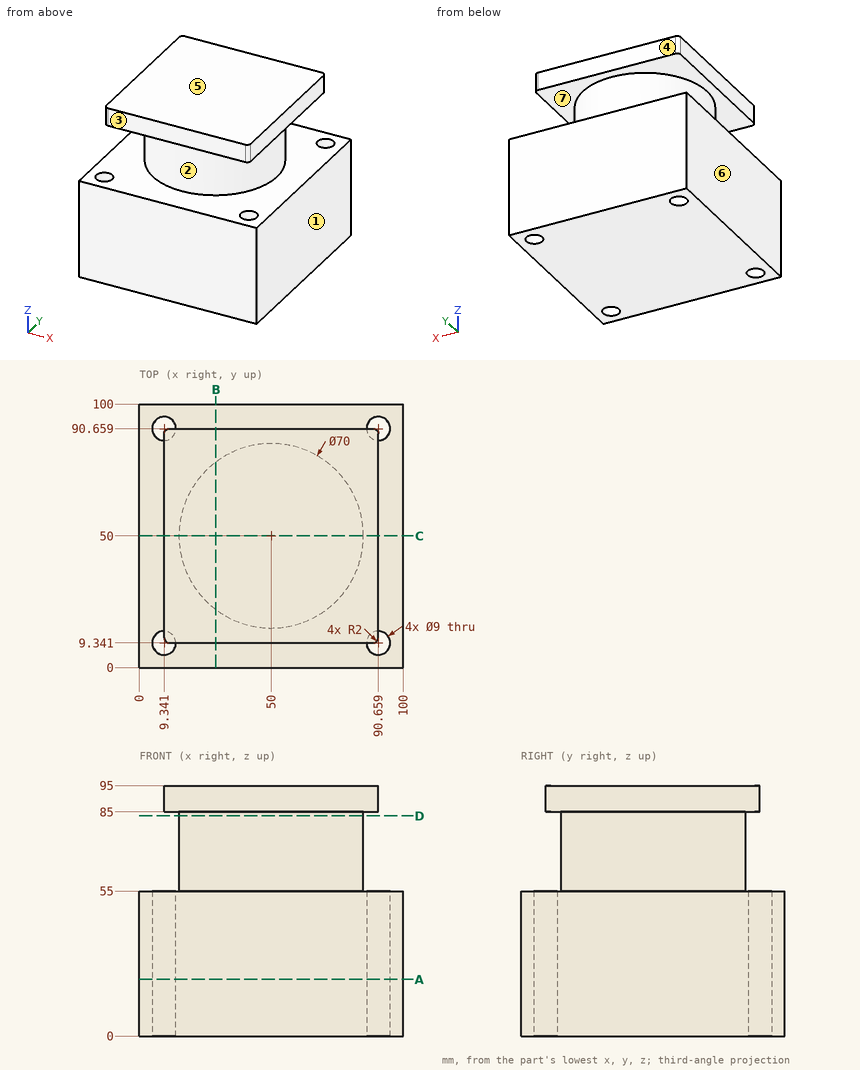
Input: dimensioned drawing with shaded views. Units: mm. Origin: part minimum x, y, z. A direction names the side the tool comes from. Round coordinates to 2 decimals unless told otherwise and drop trailing zeros. Order: outer loops, then holes, each group sorted by start corner. A loop starts at its lowest first (then second) coordinate and runs counter-clockwise, first axis right, second up. Notation, with made-up numbers: (87.5, 2) - (95.5, 2) arc R20 cw to (95.5, 8) - close; hole circle Ø10 at (-35, 55). An arc over 180 degrees is marked (long way). Use CSV: the item, a comma, the result in double quotes. Start each with the question number.
Q1. Material intervals for line 1 along X through (y, z) = (88, 42); line 2 along Z through (x, y) = (82.5, 88); line 3 along Y through (x, z) = (90, 19), sorted ascending. Write a range as from..to.
Q2. Section query B-B (x = 29). Return loops of the section in (y, z).
Q3. Mould query, pull axis Z, two halves, no side actions, for the marked faces 5, 6 and 7. Classes: +Z half, -Z half, draft (parallel to the pull), parting line (faces both ways), or undercut.
Q4. Section query A-A (z = 21.5). Return loops of the section in (x, y).
Q5. Access query for the marked faces 1, 2, 3 and 4. Directions: +Z, -Z, +X, -X, +Y, -Y. A direction counts if a zero-diameter tool reaches every point of the face in a straight line with its end or side. Return the directions, or none.
Q6. Section query C-C (y = 50). Return loops of the section in (x, z).
Q7. Section query D-D (z = 83.5). Return loops of the section in (x, y).
Q8. First-contact query: pin 1 (1 mm diameter, centred on x = 42.5, y = 29.5, fed in from -Z); pin 2 (5 mm diameter, centred on y = 35, z = 92.5, fed in from +X); pin 3 (5 mm diameter, centred on x = 21.5, z = 67.5, fed in from -Y); pin 4 (8 mm diameter, centred on y = 31.5, z = 92, fed in from -X). Flat tips, straight axial feed; report the tip coordinate or a pass-through.
Result set:
1,line 1,"x = 0..5.71, 12.97..87.03, 94.29..100"
1,line 2,"z = 0..55, 85..95"
1,line 3,"y = 0..4.89, 13.79..86.21, 95.11..100"
2,outline,"(0, 0) - (100, 0) - (100, 55) - (78, 55) - (78, 85) - (90.66, 85) - (90.66, 95) - (9.34, 95) - (9.34, 85) - (22, 85) - (22, 55) - (0, 55) - close"
3,face 5,"+Z half"
3,face 6,"draft"
3,face 7,"undercut"
4,outline,"(0, 0) - (100, 0) - (100, 100) - (0, 100) - close; hole circle Ø9 at (9.34, 9.34); hole circle Ø9 at (9.34, 90.66); hole circle Ø9 at (90.66, 9.34); hole circle Ø9 at (90.66, 90.66)"
5,face 1,"+Z, -Z, +X, +Y, -Y"
5,face 2,"none"
5,face 3,"+Z, +X, -X, -Y"
5,face 4,"+Z, +X, -X, +Y"
6,outline,"(0, 0) - (100, 0) - (100, 55) - (85, 55) - (85, 85) - (90.66, 85) - (90.66, 95) - (9.34, 95) - (9.34, 85) - (15, 85) - (15, 55) - (0, 55) - close"
7,outline,"circle Ø70 at (50, 50)"
8,pin 1,"stops at z = 0"
8,pin 2,"stops at x = 90.66"
8,pin 3,"stops at y = 26.57"
8,pin 4,"stops at x = 9.34"
